```python
from build123d import *

# Parameters (mm, degrees)
SKETCH1_R           = 127
BOSS_EXTRUDE1_DEPTH = 19.05
SKETCH2_R           = 127
SKETCH2_R_2         = 120.65
CUT_EXTRUDE1_DEPTH  = 12.7
FILLET1_R           = 1.524
SKETCH3_R           = 120.65
SKETCH3_R_2         = 117.475
CUT_EXTRUDE2_DEPTH  = 1.5875
LPATTERN1_COUNT     = 3
LPATTERN1_PITCH     = 6.35
LPATTERN1_COL_COUNT = 3
LPATTERN1_COL_PITCH = 6.35
CUT_EXTRUDE3_DEPTH  = 101.6


with BuildPart() as part:
    # Sketch1 → Boss-Extrude1 (new, symmetric)
    with BuildSketch(Plane.XY):
        with Locations(Location((0, 0, 0), (0, 0, 180))):
            Circle(SKETCH1_R)
    extrude(amount=BOSS_EXTRUDE1_DEPTH, both=True)

    # Sketch2 → Cut-Extrude1 (cut, symmetric)
    with BuildSketch(Plane.XY):
        with Locations(Location((0, 0, 0), (0, 0, 180))):
            Circle(SKETCH2_R)
        Circle(SKETCH2_R_2, mode=Mode.SUBTRACT)
    extrude(amount=CUT_EXTRUDE1_DEPTH, both=True, mode=Mode.SUBTRACT)

    # Fillet1
    fillet1_edges = [part.edges().sort_by_distance(p)[0] for p in [
        (127, 0, -19.05),
        (127, 0, 19.05),
        (127, 0, -12.7),
        (127, 0, 12.7),
    ]]
    fillet(fillet1_edges, radius=FILLET1_R)

    # Sketch3 → Cut-Extrude2 (cut, symmetric)
    with BuildSketch(Plane.XY):
        Circle(SKETCH3_R)
        Circle(SKETCH3_R_2, mode=Mode.SUBTRACT)
    cut_extrude2 = extrude(amount=CUT_EXTRUDE2_DEPTH, both=True, mode=Mode.SUBTRACT)

    # LPattern1: Cut-Extrude2 ×3
    with Locations(*[(0, 0, -i * LPATTERN1_PITCH) for i in range(1, LPATTERN1_COUNT)]):
        add(cut_extrude2, mode=Mode.SUBTRACT)

    # LPattern1 col: Cut-Extrude2 ×3
    with Locations(*[(0, 0, i * LPATTERN1_COL_PITCH) for i in range(1, LPATTERN1_COL_COUNT)]):
        add(cut_extrude2, mode=Mode.SUBTRACT)

    # Sketch4 → Cut-Extrude3 (cut)
    with BuildSketch(Plane.XY.offset(19.05)):
        with BuildLine():
            Line((-3.175, 22.225), (3.175, 22.225))
            Line((3.175, 22.225), (3.175, 15.554259867))
            ThreePointArc((3.175, 15.554259867), (0, -15.875), (-3.175, 15.554259867))
            Line((-3.175, 15.554259867), (-3.175, 22.225))
        make_face()
    extrude(amount=-CUT_EXTRUDE3_DEPTH, mode=Mode.SUBTRACT)


solid = part.part
```
Read the model definition and answer for the solid it produces. Units are mm, in the model's axes. A direction names the side the tool comes from. Coordinates: 2 decimals unless noted, no trailing zeros. Answer as a JSON object with one key per item and string values. Group by question number.
Item 1: Consider probe 1 along Y at (x, z) = (0, -13.45) (3 decimals); probe 2 along Y at (x, z) = (0, -4) (3 decimals); probe 3 along Y at (x, z) = (0, 13) (3 decimals). Determine where each line is inside the solid, lowest interval first. Write a range as from..to.
Item 2: Flat-ended cylindrical pins translate along their axes: P1, Ø4, axis at x = -92, z = 4.5, coming from the -Y side; P2, Ø3, axis at x = -83.5, z = -11.5, coming from the -Y side; P3, Ø3, axis at x = 10, z = 13, coming from the +Y side. Find the tip coordinate at first contact, or state that the pin passes through.
Item 3: A tool of negligible diameter and unlimited length cuts with its end or side. For faces 5 (the face through (26, -116, -4.762)), 6 (the face through (3.175, 19, 0)), from which of +Z, -Z, +X, -X, +Y, -Y can it reach the whole face along a straight path? Write none if from no direction.
Item 4: The mould has two halves that part along Z. Classify faces 1 (the face through (26, -116, 4.762)), 2 (the face through (0.65, -15.86, 0.27)), 3 (the face through (-120.533, 5.305, 13.505)), 4 (the face through (2, 26, -19.05)): +Z half, -Z half, draft (parallel to the pull), parting line (faces both ways), or undercut.
Results are:
{
 "1": {"probe 1": "y = -126.789..-120.65, -117.475..-15.875, 22.225..117.475, 120.65..126.789", "probe 2": "y = -120.65..-15.875, 22.225..120.65", "probe 3": "y = -126.384..-120.65, -117.475..-15.875, 22.225..117.475, 120.65..126.384"},
 "2": {"P1": "stops at y = -80.35", "P2": "stops at y = -95.14", "P3": "stops at y = 126.68"},
 "3": {"face 5": "none", "face 6": "+Z, -Z"},
 "4": {"face 1": "undercut", "face 2": "draft", "face 3": "undercut", "face 4": "-Z half"}
}
